Here's how the part is built. I have some questions about the finished solid (model axes, mm). A direction names the side the tool comes from. Coordinates: 2 decimals unless noted, no trailing zeros. Write each loop counter-clockwise with the first axis right and the second up, starting at its lowest first coordinate (ties: lowest second). Pieces come first, ordered by that corner, then holes. Notation, with made-up numbers: (1, 20.5) -> (48, 20.5) arc R29 cw to (48, 40.5) -> close; hole circle Ø8 at (-4, -29.75). An arc over 180 degrees is marked (long way). Put each result on its own line as item: value.
```python
from build123d import *

# Parameters (mm, degrees)
SKETCH1_W            = 26
SKETCH1_H            = 46
SKETCH1_W_2          = 20.5
SKETCH1_H_2          = 40.5
BOSS_EXTRUDE1_DEPTH  = 26
SKETCH2_W            = 26
SKETCH2_H            = 46
BOSS_EXTRUDE2_DEPTH  = 2
SKETCH3_W            = 7
SKETCH3_H            = 3
CUT_EXTRUDE1_DEPTH   = 22
SKETCH6_W            = 3
SKETCH6_H            = 40
BOSS_EXTRUDE5_DEPTH  = 7
SKETCH7_W            = 3
SKETCH7_H            = 40
BOSS_EXTRUDE6_DEPTH  = 7
SKETCH8_W            = 46
SKETCH8_H            = 12
BOSS_EXTRUDE7_DEPTH  = 3
SKETCH10_W           = 23.5
SKETCH10_H           = 60
BOSS_EXTRUDE8_DEPTH  = 3
SKETCH11_W           = 60
SKETCH11_H           = 43
BOSS_EXTRUDE9_DEPTH  = 3
BOSS_EXTRUDE10_DEPTH = 40
BOSS_EXTRUDE11_DEPTH = 40


with BuildPart() as part:
    # Sketch1 → Boss-Extrude1 (new body)
    with BuildSketch(Plane(origin=(0, 0, 0), x_dir=(1, 0, 0), z_dir=(0, 1, 0))):
        Rectangle(SKETCH1_W, SKETCH1_H)
        Rectangle(SKETCH1_W_2, SKETCH1_H_2, mode=Mode.SUBTRACT)
    extrude(amount=BOSS_EXTRUDE1_DEPTH)

    # Sketch2 → Boss-Extrude2 (add)
    with BuildSketch(Plane(origin=(0, 26, 0), x_dir=(1, 0, 0), z_dir=(0, 1, 0))):
        Rectangle(SKETCH2_W, SKETCH2_H)
    extrude(amount=BOSS_EXTRUDE2_DEPTH)

    # Sketch3 → Cut-Extrude1 (cut)
    with BuildSketch(Plane.XZ):
        with Locations((0, 21.5)):
            Rectangle(SKETCH3_W, SKETCH3_H)
    extrude(amount=-CUT_EXTRUDE1_DEPTH, mode=Mode.SUBTRACT)

    # Sketch6 → Boss-Extrude5 (add)
    with BuildSketch(Plane.XY.offset(23)):
        with Locations((-11.5, 20)):
            Rectangle(SKETCH6_W, SKETCH6_H)
    extrude(amount=BOSS_EXTRUDE5_DEPTH)

    # Sketch7 → Boss-Extrude6 (add)
    with BuildSketch(Plane(origin=(0, 0, -23), x_dir=(-1, 0, 0), z_dir=(0, 0, -1))):
        with Locations((11.5, 20)):
            Rectangle(SKETCH7_W, SKETCH7_H)
    extrude(amount=BOSS_EXTRUDE6_DEPTH)

    # Sketch8 → Boss-Extrude7 (add)
    with BuildSketch(Plane(origin=(-10, 0, 0), x_dir=(0, 0, -1), z_dir=(1, 0, 0))):
        with Locations((0, 34)):
            Rectangle(SKETCH8_W, SKETCH8_H)
    extrude(amount=-BOSS_EXTRUDE7_DEPTH)

    # Sketch10 → Boss-Extrude8 (add)
    with BuildSketch(Plane(origin=(0, 40, 0), x_dir=(1, 0, 0), z_dir=(0, 1, 0))):
        with Locations((-21.75, 0)):
            Rectangle(SKETCH10_W, SKETCH10_H)
    extrude(amount=BOSS_EXTRUDE8_DEPTH)

    # Sketch11 → Boss-Extrude9 (add)
    with BuildSketch(Plane.ZY.offset(33.5)):
        with Locations((0, 21.5)):
            Rectangle(SKETCH11_W, SKETCH11_H)
    extrude(amount=BOSS_EXTRUDE9_DEPTH)

    # Sketch12 → Boss-Extrude10 (add)
    with BuildSketch(Plane.XY.offset(30)):
        Polygon((-33.5, 0), (-36.5, 0), (-36.5, 43), (-10, 43), (-10, 0), (-13, 0), (-13, 40), (-33.5, 40), align=None)
    extrude(amount=BOSS_EXTRUDE10_DEPTH)

    # Sketch13 → Boss-Extrude11 (add)
    with BuildSketch(Plane(origin=(0, 0, -30), x_dir=(-1, 0, 0), z_dir=(0, 0, -1))):
        Polygon((13, 0), (10, 0), (10, 43), (36.5, 43), (36.5, 0), (33.5, 0), (33.5, 40), (13, 40), align=None)
    extrude(amount=BOSS_EXTRUDE11_DEPTH)


solid = part.part
```
Item 1: If we mould it in two halves opening along X, with no side actions, what happens to faces 4 (the flat face through (13, 14, 0)), 5 (the flat face through (-36.5, 22, 1)), 6 (the flat face through (0, 22, 22)), 7 (the flat face through (-34, 26, -70))? For each: released by +X, released by -X, zero draft, split by the parting line, or undercut.
Output:
face 4: released by +X
face 5: released by -X
face 6: undercut
face 7: zero draft
Item 2: Which directions (+Z, -Z, +X, -X, +Y, -Y) give clear straight access to the entire face, cutting with the end or side of a thin tool? Please do faces 1 (the flat face through (1, 14, -23)), 2 (the flat face through (-13, 20, 1)), 3 (the flat face through (-10.25, 13, 0)).
Output:
face 1: -Z, +X, +Y, -Y
face 2: +Z, -Z, -Y
face 3: -Y
Item 3: Please list where these lines run through material, in increasing order: line 1 along X through (y, z) = (17.5, -12.5); line 2 along X through (y, z) = (14, 32.5); line 3 along Z through (x, y) = (7, 7.5). Write a range as from..to.
Output:
line 1: x = -36.5..-33.5, -13..-10.25, 10.25..13
line 2: x = -36.5..-33.5, -13..-10
line 3: z = -23..-20.25, 20.25..23
Item 4: Imagine slicing it at C-C on z = -4.5. Write out the boundary of the cut face in (x, y).
Output:
outline: (-36.5, 0) -> (-33.5, 0) -> (-33.5, 40) -> (-13, 40) -> (-13, 0) -> (-10.25, 0) -> (-10.25, 26) -> (10.25, 26) -> (10.25, 0) -> (13, 0) -> (13, 28) -> (-10, 28) -> (-10, 43) -> (-36.5, 43) -> close
Item 5: Imagine slicing it at B-B on x = 2. Write out the boundary of the cut face in (y, z), then the cut area to 4 significant figures.
Output:
outline: (0, -23) -> (28, -23) -> (28, 23) -> (22, 23) -> (22, 20.25) -> (26, 20.25) -> (26, -20.25) -> (0, -20.25) -> close
area: 174.5 mm²
Item 6: For P1, Ø8, axis at x = -15.5, y = 17.5, coming from the +Z side; P2, Ø16.5, axis at x = 0.5, y = 15.5, coming from the +Z side; P3, Ø0.8, axis at x = 0.5, z = 21, coming from the -Y side; P4, Ø10, axis at x = -4, z = -9.5, coming from the -Y side, each with a flat end and sliding along its axis, tell me the tip position at first contact or that it passes through.
Output:
P1: stops at z = 70
P2: stops at z = 23
P3: stops at y = 22
P4: stops at y = 26
Item 7: Imagine slicing it at A-A on y = 15. Write out the boundary of the cut face in (x, z), then the cut area to 3 significant figures.
Output:
outline: (-36.5, -70) -> (-33.5, -70) -> (-33.5, 70) -> (-36.5, 70) -> close; (-13, -70) -> (-10, -70) -> (-10, -23) -> (13, -23) -> (13, 23) -> (3.5, 23) -> (3.5, 20.25) -> (10.25, 20.25) -> (10.25, -20.25) -> (-10.25, -20.25) -> (-10.25, 20.25) -> (-3.5, 20.25) -> (-3.5, 23) -> (-10, 23) -> (-10, 70) -> (-13, 70) -> close
area: 1,050 mm²
Item 8: Imagine slicing it at D-D on y = 35. Write out the boundary of the cut face in (x, z), then the cut area to 3 significant figures.
Output:
outline: (-36.5, -70) -> (-33.5, -70) -> (-33.5, 70) -> (-36.5, 70) -> close; (-13, -70) -> (-10, -70) -> (-10, 70) -> (-13, 70) -> close
area: 840 mm²
